from build123d import *

# Parameters (mm, degrees)
BOSS_EXTRUDE1_DEPTH  = 6
FILLET1_R            = 5
SKETCH2_R            = 2.25
SKETCH2_R_2          = 1.6
CUT_EXTRUDE1_DEPTH   = 89.662280593
FILLET1_OF_MIRROR1_R = 5


with BuildPart() as part:
    # Sketch1 → Boss-Extrude1 (new body)
    with BuildSketch(Plane(origin=(0, 0, 0), x_dir=(1, 0, 0), z_dir=(0, 1, 0))):
        Polygon((0, 0), (-50, 0), (-50, 60), (-65, 60), (-65, -15), (0, -15), align=None)
    boss_extrude1 = extrude(amount=BOSS_EXTRUDE1_DEPTH)

    # Fillet1
    fillet1_edges = [part.edges().sort_by_distance(p)[0] for p in [
        (-65, 3, 15),
        (-65, 3, -60),
        (-50, 3, -60),
        (-50, 3, 0),
    ]]
    fillet(fillet1_edges, radius=FILLET1_R)

    # Sketch2 → Cut-Extrude1 (cut, through all)
    with BuildSketch(Plane(origin=(0, 6, 0), x_dir=(1, 0, 0), z_dir=(0, 1, 0))):
        with Locations(Location((-15, -7.5, 0), (0, 0, 270))):
            Circle(SKETCH2_R)
        with Locations(Location((-45, -7.5, 0), (0, 0, 270))):
            Circle(SKETCH2_R_2)
        with Locations(Location((-57.5, 55, 0), (0, 0, 270))):
            Circle(SKETCH2_R_2)
        with Locations(Location((-57.5, 25, 0), (0, 0, 270))):
            Circle(SKETCH2_R_2)
    cut_extrude1 = extrude(amount=-CUT_EXTRUDE1_DEPTH, mode=Mode.SUBTRACT)

    # Mirror1: Boss-Extrude1, Cut-Extrude1 across plane
    add(boss_extrude1.mirror(Plane(origin=(0, 0, 0), x_dir=(0, 0, 1), z_dir=(1, 0, 0))))
    add(cut_extrude1.mirror(Plane(origin=(0, 0, 0), x_dir=(0, 0, 1), z_dir=(1, 0, 0))), mode=Mode.SUBTRACT)

    # Fillet1 of Mirror1
    fillet1_of_mirror1_edges = [part.edges().sort_by_distance(p)[0] for p in [
        (65, 3, 15),
        (65, 3, -60),
        (50, 3, -60),
        (50, 3, 0),
    ]]
    fillet(fillet1_of_mirror1_edges, radius=FILLET1_OF_MIRROR1_R)


solid = part.part
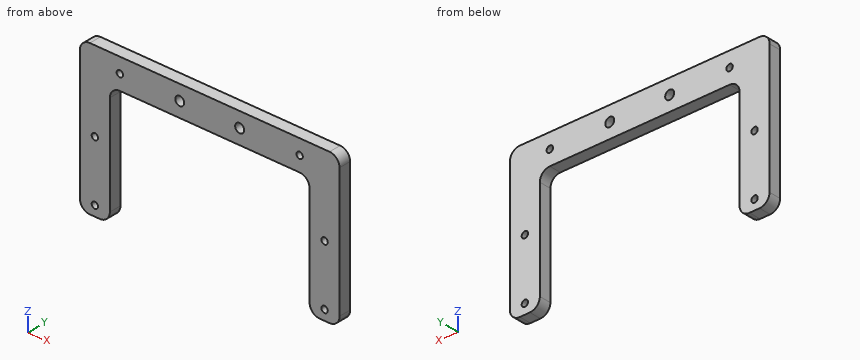
Work out the finished part from the listing and answer in its coordinate system (mm). Give positions to 0.01 mm unless a question says otherwise; leave off trailing zeros. Order: outer loops, then holes, each group sorted by start corner. A loop starts at its lowest first (then second) coordinate and runs counter-clockwise, first axis right, second up. Notation, with made-up numbers: (-36, 64.5) -> (-28, 64.5) arc R16 ccw to (-28, 74.5) -> close; hole circle Ø9 at (-15, 76.25). An arc over 180 degrees is marked (long way). Answer as a JSON object with one key per item and string values. Group by question number.
1. Section C-C on z = -47 is taken. Determine the outline of the cut face in (x, y).
2. Section B-B on y = 1.55 is taken. Count the separate pieces of the cut face and the enclosed holes in it, plus the area to 3 significant figures.
3. Section D-D on x = 33.5 is taken. Determine the outline of the cut face in (y, z), plus the area to 3 significant figures.
4. Consider line 1 along X through (y, z) = (3.2, -25); line 2 along X through (y, z) = (2.8, 7.5); line 3 along X through (y, z) = (3.8, -24). Determine where each line is inside the solid, lowest interval first. Write a range as [from, to].
5. Section A-A on x = 57.5 is taken. Determine the outline of the cut face in (y, z), plus the area to 3 significant figures.
6. Flat-ended cylindrical pins translate along their axes: pin 1 Ø3.5 at (x, z) = (-15, 7.5) entering from -Y; pin 2 Ø2 at (x, y) = (-5, 3.5) entering from -Z. Find the tip coordinate at first contact, or state that the pin passes through.
Result sheet:
{
 "1": {"outline": "(-65, 0) -> (-50, 0) -> (-50, 6) -> (-65, 6) -> close; (50, 0) -> (65, 0) -> (65, 6) -> (50, 6) -> close"},
 "2": {"separate pieces": "1", "enclosed holes": "8", "area": "3,650 mm^2"},
 "3": {"outline": "(0, 0) -> (6, 0) -> (6, 15) -> (0, 15) -> close", "area": "90.0 mm^2"},
 "4": {"line 1": "x = [-65, -59.1], [-55.9, -50], [50, 55.9], [59.1, 65]", "line 2": "x = [-65, -46.6], [-43.4, -17.25], [-12.75, 12.75], [17.25, 43.4], [46.6, 65]", "line 3": "x = [-65, -58.75], [-56.25, -50], [50, 56.25], [58.75, 65]"},
 "5": {"outline": "(0, -60) -> (6, -60) -> (6, -56.6) -> (0, -56.6) -> close; (0, -53.4) -> (6, -53.4) -> (6, -26.6) -> (0, -26.6) -> close; (0, -23.4) -> (6, -23.4) -> (6, 15) -> (0, 15) -> close", "area": "412 mm^2"},
 "6": {"pin 1": "passes through", "pin 2": "stops at z = 0"}
}
